from build123d import *

# Parameters (mm, degrees)
SKETCH_W        = 97
SKETCH_H        = 54
PAD_DEPTH       = 24
SKETCH001_W     = 93
SKETCH001_H     = 50
POCKET_DEPTH    = 19
SKETCH002_R     = 1.8
POCKET001_DEPTH = 24.001
SKETCH003_R     = 3.2
POCKET002_DEPTH = 3
SKETCH004_W     = 67
SKETCH004_H     = 2
SKETCH004_W_2   = 2
SKETCH004_H_2   = 24
PAD001_DEPTH    = 5
SKETCH005_W     = 13
SKETCH005_H     = 9
POCKET003_DEPTH = 2
SKETCH006_W     = 12
SKETCH006_H     = 14
POCKET004_DEPTH = 2
FILLET_R        = 2
SKETCH007_W     = 10
SKETCH007_H     = 10
POCKET005_DEPTH = 16
SKETCH008_W     = 3
SKETCH008_H     = 5
POCKET006_DEPTH = 5.001
FILLET001_R     = 1


with BuildPart() as part:
    # Sketch → Pad (new body)
    with BuildSketch(Plane.XY):
        with Locations((48.5, 27)):
            Rectangle(SKETCH_W, SKETCH_H)
    extrude(amount=PAD_DEPTH)

    # Sketch001 → Pocket (cut)
    with BuildSketch(Plane.XY.offset(24)):
        with Locations((48.5, 27)):
            Rectangle(SKETCH001_W, SKETCH001_H)
    extrude(amount=-POCKET_DEPTH, mode=Mode.SUBTRACT)

    # Sketch002 → Pocket001 (cut, through all)
    with BuildSketch(Plane(origin=(0, 0, 0), x_dir=(1, 0, 0), z_dir=(0, 0, -1))):
        with Locations((6, -5.5)):
            Circle(SKETCH002_R)
        with Locations((91, -5.5)):
            Circle(SKETCH002_R)
        with Locations((91, -48.5)):
            Circle(SKETCH002_R)
        with Locations((6, -48.5)):
            Circle(SKETCH002_R)
    extrude(amount=-POCKET001_DEPTH, mode=Mode.SUBTRACT)

    # Sketch003 → Pocket002 (cut)
    with BuildSketch(Plane(origin=(0, 0, 0), x_dir=(1, 0, 0), z_dir=(0, 0, -1))):
        with Locations((6, -5.5)):
            Circle(SKETCH003_R)
        with Locations((6, -48.5)):
            Circle(SKETCH003_R)
        with Locations((91, -5.5)):
            Circle(SKETCH003_R)
        with Locations((91, -48.5)):
            Circle(SKETCH003_R)
    extrude(amount=-POCKET002_DEPTH, mode=Mode.SUBTRACT)

    # Sketch004 → Pad001 (new body)
    with BuildSketch(Plane.XY.offset(5)):
        with Locations((48.5, 3)):
            Rectangle(SKETCH004_W, SKETCH004_H)
        with Locations((48.5, 51)):
            Rectangle(SKETCH004_W, SKETCH004_H)
        with Locations((3, 27)):
            Rectangle(SKETCH004_W_2, SKETCH004_H_2)
        with Locations((94, 27)):
            Rectangle(SKETCH004_W_2, SKETCH004_H_2)
    extrude(amount=PAD001_DEPTH)

    # Sketch005 → Pocket003 (cut)
    with BuildSketch(Plane.XZ):
        with Locations((26.5, 19.5)):
            Rectangle(SKETCH005_W, SKETCH005_H)
    extrude(amount=-POCKET003_DEPTH, mode=Mode.SUBTRACT)

    # Sketch006 → Pocket004 (cut)
    with BuildSketch(Plane.XZ):
        with Locations((80, 17)):
            Rectangle(SKETCH006_W, SKETCH006_H)
    extrude(amount=-POCKET004_DEPTH, mode=Mode.SUBTRACT)

    # Fillet
    fillet_edges = [part.edges().sort_by_distance(p)[0] for p in [
        (97, 0, 12),
        (0, 0, 12),
        (97, 54, 12),
        (0, 54, 12),
    ]]
    fillet(fillet_edges, radius=FILLET_R)

    # Sketch007 → Pocket005 (cut)
    with BuildSketch(Plane.XY.offset(24)):
        with Locations((6.6, 6.6)):
            Rectangle(SKETCH007_W, SKETCH007_H)
        with Locations((6.6, 47.4)):
            Rectangle(SKETCH007_W, SKETCH007_H)
        with Locations((90.4, 6.6)):
            Rectangle(SKETCH007_W, SKETCH007_H)
        with Locations((90.4, 47.4)):
            Rectangle(SKETCH007_W, SKETCH007_H)
    extrude(amount=-POCKET005_DEPTH, mode=Mode.SUBTRACT)

    # Sketch008 → Pocket006 (cut, through all)
    with BuildSketch(Plane.XY.offset(5)):
        with Locations((7.5, 27)):
            Rectangle(SKETCH008_W, SKETCH008_H)
    extrude(amount=-POCKET006_DEPTH, mode=Mode.SUBTRACT)

    # Fillet001
    fillet001_edges = [part.edges().sort_by_distance(p)[0] for p in [
        (6, 27, 5),
        (9, 27, 5),
        (7.5, 29.5, 5),
        (7.5, 24.5, 5),
    ]]
    fillet(fillet001_edges, radius=FILLET001_R)


solid = part.part
Model file for the job. Use its own axes, mm. A direction names the side the tool comes from. Give positions to 0.01 mm unless a question says otherwise; leave off trailing zeros. Loops run counter-clockwise (first coordinate to the right, second up) from the corner with the lowest first, then second, coordinate; pieces in that order, holes last.
1) Saw through at D-D (z = 6.75). Write the cut outline in (x, y).
2) Wall check: line 1 (Y direction, x = 91, z = 4.65); line 2 (X direction, y = 48.5, z = 3.85); line 3 (Y direction, x = 91, z = 1.8). Give the ranges that are in metal, low to high.
3) Flat gauge pins, fed straight in: pin 1 Ø3 at (x, y) = (7.5, 48.5) entering from +Z; pin 2 Ø1 at (y, z) = (1, 14) entering from +X; pin 3 Ø4 at (x, y) = (91, 48.5) entering from -Z. Where does each tip first touch, or does it go through?
4) Pull direction X, two halves, no side cores. Call faces 4 (the cylindrical face through (3.461, 7.447, 1.479)), 5 (the cylindrical face through (96.4, 53.43, 12.17)), 6 (the flat face through (48, 0, 12)): +X half, -X half, draft (parallel to the pull), parting line (faces both ways), or undercut.
5) Saw through at A-A (y = 5.5). Write the cut outline in (x, z).
6) Saw through at B-B (x = 91). Write the cut outline in (y, z).
7) Tool access for faces 1 (the flat face through (6, 27, 2)), 2 (the flat face through (1.8, 4.4, 8)), 3 (the flat face through (20, 1, 19)): list every direction of +Z, -Z, +X, -X, +Y, -Y with a clear straight run to the whole face (end or side of a thin tool).
Answer block:
1. outline: (0, 2) arc R2 ccw to (2, 0) - (95, 0) arc R2 ccw to (97, 2) - (97, 52) arc R2 ccw to (95, 54) - (2, 54) arc R2 ccw to (0, 52) - close; hole (2, 2) - (15, 2) - (15, 4) - (82, 4) - (82, 2) - (95, 2) - (95, 15) - (93, 15) - (93, 39) - (95, 39) - (95, 52) - (82, 52) - (82, 50) - (15, 50) - (15, 52) - (2, 52) - (2, 39) - (4, 39) - (4, 15) - (2, 15) - close
2. line 1: y = 0 to 3.7, 7.3 to 46.7, 50.3 to 54
2. line 2: x = 0 to 4.2, 7.8 to 89.2, 92.8 to 97
2. line 3: y = 0 to 2.3, 8.7 to 45.3, 51.7 to 54
3. pin 1: stops at z = 5
3. pin 2: stops at x = 96.94
3. pin 3: stops at z = 3
4. face 4: undercut
4. face 5: +X half
4. face 6: draft
5. outline: (0, 0) - (2.8, 0) - (2.8, 3) - (4.2, 3) - (4.2, 5) - (2, 5) - (2, 8) - (1.6, 8) - (1.6, 24) - (0, 24) - close; (7.8, 3) - (9.2, 3) - (9.2, 0) - (87.8, 0) - (87.8, 3) - (89.2, 3) - (89.2, 5) - (7.8, 5) - close; (92.8, 3) - (94.2, 3) - (94.2, 0) - (97, 0) - (97, 24) - (95.4, 24) - (95.4, 8) - (95, 8) - (95, 5) - (92.8, 5) - close
6. outline: (0, 0) - (2.3, 0) - (2.3, 3) - (3.7, 3) - (3.7, 5) - (2, 5) - (2, 8) - (1.6, 8) - (1.6, 24) - (0, 24) - close; (7.3, 3) - (8.7, 3) - (8.7, 0) - (45.3, 0) - (45.3, 3) - (46.7, 3) - (46.7, 5) - (7.3, 5) - close; (50.3, 3) - (51.7, 3) - (51.7, 0) - (54, 0) - (54, 24) - (52.4, 24) - (52.4, 8) - (52, 8) - (52, 5) - (50.3, 5) - close
7. face 1: +Z, -Z
7. face 2: +Z
7. face 3: +Z, -Y
